Can you work these out from the drawing? Everything is in mm from the part's minimum corner. A direction names the side the tool comes from. Give positions to 0.01 mm unless a question says otherwise; leave off trailing zeros. Loops run counter-clockwise (first coordinate to the right, second up) from the corner with the lowest first, then second, coordinate; pieces in that order, holes last. Notation, with made-up numbers: (22, 22) - (44, 22) arc R29 ccw to (44, 49) - close; hole circle Ø7 at (-34.75, 55.25). An arc over 180 degrees is marked (long way). One line per item, written item: value. Start each with the question number.
Q1. For the marked faces 4, 5, 6, 7 and 8, which set-ups out of +Z, -Z, +X, -X, +Y, -Y let a thin tool reach every point of the face, with its end or its side?
Q2. I want a section at C-C (z = 0.6). Please give me the cut outline in (x, y), then the cut area to 3 significant figures.
Q3. If we mould it in two halves opening along Z, with no side actions, what happens to the marked faces 1, 2 and 3? For each: released by +Z, released by -Z, zero draft, split by the parting line, or undercut.
Q4. I want a section at A-A (y = 2.55). Please give me the cut outline in (x, z), then the cut area to 3 significant figures.
Q5. I want a section at B-B (x = 2). Please give me the cut outline in (y, z), then the cut area to 3 significant figures.
Q6. If I drill on line 1 (Y direction, x = 4.25, z = 2.3); line 2 (Y direction, x = 3.25, z = 3.7), over which ranges is the centre line in solid material (lowest first)? Write a range as from..to.
Q7. I want a section at D-D (y = 3.55). Please give me the cut outline in (x, z).
Q8. I'm going to push flat-ended pins straight in: P1, Ø0.5, axis at x = 2.5, z = 3.5, coming from the +Y side; P2, Ø0.5, axis at x = 4, y = 2.5, coming from the -Z side; P3, Ø1.1, axis at y = 3.5, z = 0.5, coming from the +X side. Where does each tip first touch, or does it pass through?
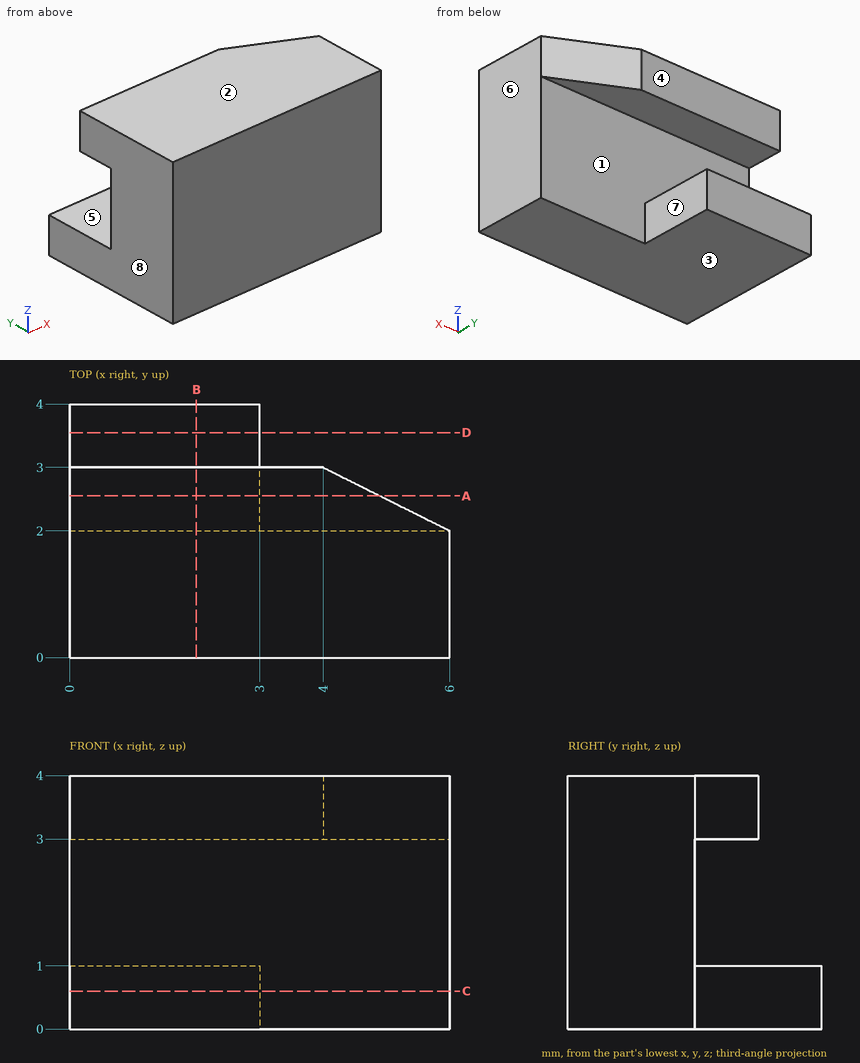
Worked answers:
1. face 4: +Z, +X, -X, +Y
1. face 5: +X, -X, +Y
1. face 6: +Z, -Z, +X, +Y, -Y
1. face 7: -Z, +X, +Y
1. face 8: +Z, -Z, -X, +Y, -Y
2. outline: (0, 0) - (6, 0) - (6, 2) - (3, 2) - (3, 4) - (0, 4) - close
2. area: 18.0 mm²
3. face 1: undercut
3. face 2: released by +Z
3. face 3: released by -Z
4. outline: (0, 0) - (3, 0) - (3, 1) - (0, 1) - close; (0, 3) - (4.9, 3) - (4.9, 4) - (0, 4) - close
4. area: 7.90 mm²
5. outline: (0, 0) - (4, 0) - (4, 1) - (2, 1) - (2, 3) - (3, 3) - (3, 4) - (0, 4) - close
5. area: 11.0 mm²
6. line 1: y = 0..2
6. line 2: y = 0..3
7. outline: (0, 0) - (3, 0) - (3, 1) - (0, 1) - close
8. P1: stops at y = 3
8. P2: stops at z = 3
8. P3: stops at x = 3
